Geometry: see drawing. Coordinates: mm, zero at the bounding-box minimum. A direction names the side the tool comes from. Give positions to 0.01 mm unless a question says otherwise; leave off trailing zeros. Order: outer loops, then holes, each group sorted by start corner. A loop starts at its lowest first (then second) coordinate and runs counter-clockwise, first axis right, second up. Notation, with made-up numbers: (89.5, 21) -> (108.5, 21) arc R17 cw to (108.5, 28) -> close; hole circle Ø11 at (48.5, 82.5). An arc over 180 degrees is marked (long way). One line per item, written item: value. Start each with the question number.
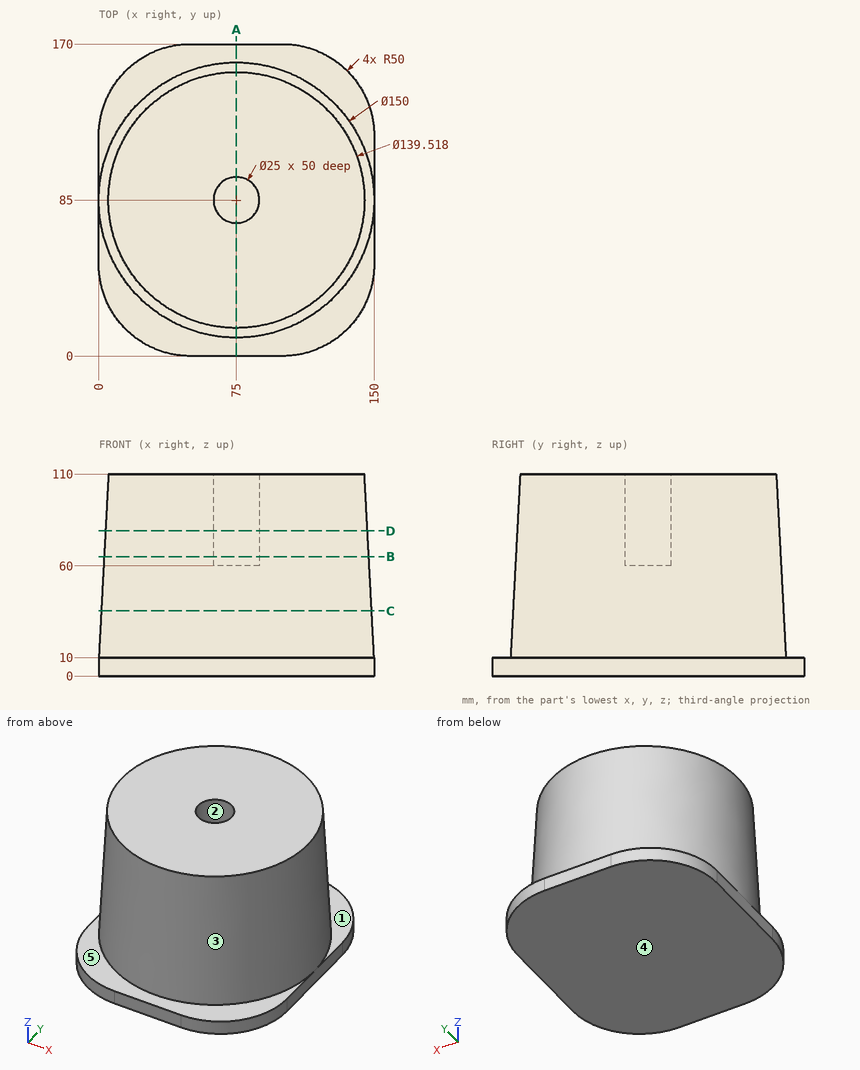
1. Cut plane B-B, the plane z = 65. Return loops of the section in (x, y) (1 decimal).
2. Cut plane D-D, the plane z = 79. Return loops of the section in (x, y).
3. Material intervals for L1, parallel to Y at x = 75, z = 83.5; L2, parallel to Y at x = 75, z = 97.5 (1 decimal); L3, parallel to Z at x = 16.5, y = 141, sorted ascending. Write a range as [from, to].
4. Pin query (flat end, axial travel): P1, Ø12, axis at y = 92.5, z = 76, coming from the +X side; P2, Ø7.5, axis at x = 79, y = 80, coming from the +Z side; P3, Ø3, axis at x = 39, z = 68.5, coming from the -Y side (1 decimal). Return the tip coordinate at first contact, or that it passes through.
5. Cut plane A-A, the plane x = 75. Return loops of the section in (y, z).
6. Cut plane C-C, the plane z = 35.5. Return loops of the section in (x, y).
7. Draft query along Y for the marked faces 1, 2 and 3. Return one class per face: pulls with the +Y half, pulls with the -Y half, needs draft (parallel to the pull), parting line crosses it, or undercut.
8. Access query for the marked faces 4 and 5. Directions: +Z, -Z, +X, -X, +Y, -Y. A direction counts if a zero-diameter tool reaches every point of the face in a straight line with its end or side. Return the directions, or none.
Answers follow:
1. outline: circle Ø144.2 at (75, 85); hole circle Ø25 at (75, 85)
2. outline: circle Ø142.77 at (75, 85); hole circle Ø25 at (75, 85)
3. L1: y = [13.85, 72.5], [97.5, 156.15]
3. L2: y = [14.6, 72.5], [97.5, 155.4]
3. L3: z = [0, 10]
4. P1: stops at x = 146.69
4. P2: stops at z = 60
4. P3: stops at y = 21.9
5. outline: (0, 0) -> (170, 0) -> (170, 10) -> (160, 10) -> (154.76, 110) -> (97.5, 110) -> (97.5, 60) -> (72.5, 60) -> (72.5, 110) -> (15.24, 110) -> (10, 10) -> (0, 10) -> close
6. outline: circle Ø147.33 at (75, 85)
7. face 1: needs draft
7. face 2: undercut
7. face 3: parting line crosses it
8. face 4: -Z, +X, -X, +Y, -Y
8. face 5: +Z, -Y
